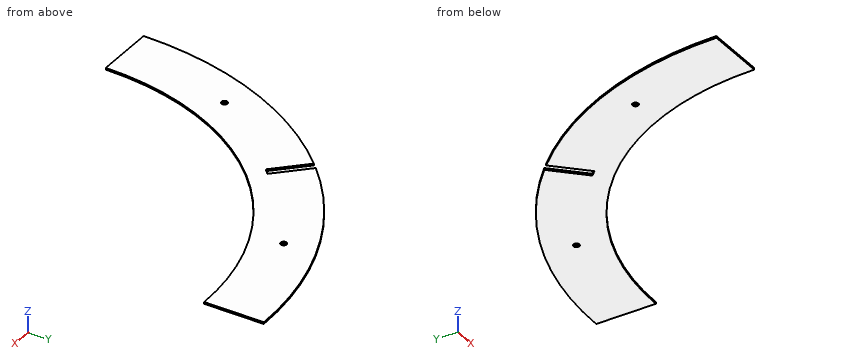
Autodesk Inventor part; units mm, degrees
ref_plane "YZ Plane" through (0, 0, 0) normal (1, 0, 0) x (0, 1, 0)
ref_plane "XZ Plane" through (0, 0, 0) normal (0, 1, 0) x (-1, 0, 0)
ref_plane "XY Plane" through (0, 0, 0) normal (0, 0, 1) x (1, 0, 0)
sketch "Sketch1" plane through (0, 0, 0) normal (0, 0, 1) x (1, 0, 0)
  arc A0 (0, 550) -> (-550, 0) centre (0, 0) ccw
  arc A1 (0, 450) -> (-450, 0) centre (0, 0) ccw
  line L0 (0, 550) -> (0, 450)
  line L1 (-450, 0) -> (-550, 0)
  point P0 (-500, 0)
  point P1 (0, 500)
  dimension "d0" = 1100
  dimension "d1" = 900
extrude "Plate1" add sketch "Sketch1" against normal blind 3
sketch "Sketch2" plane through (0, 0, 0) normal (0, 0, 1) x (1, 0, 0)
  line L0 (-550, 0) -> (-450, 0)
  arc A0 (0, 550) -> (-550, 0) centre (0, 0) ccw
  circle A1 centre (-461.9398, 191.3417) radius 5
  arc A2 (0, 450) -> (-450, 0) centre (0, 0) ccw
  line L1 (-415.7458, 172.2075) -> (-508.1337, 210.4759) construction
  point P0 (-461.9398, 191.3417)
  dimension "d4" = 10
  dimension "d5" = 22.5
extrude "Cut1" cut sketch "Sketch2" against normal through all
pattern_circular "Circular Pattern1" count 2 over 45 about axis through (0, 0, 0) along (0, 0, -1) of "Cut1"
sketch "Sketch3" plane through (0, 0, 0) normal (0, 0, 1) x (1, 0, 0)
  line L0 (-388.9087, 388.9087) -> (-318.1981, 318.1981) construction
  arc A0 (0, 450) -> (-450, 0) centre (0, 0) ccw
  arc A1 (0, 550) -> (-550, 0) centre (0, 0) ccw
  line L1 (-550, 0) -> (-450, 0)
  line L2 (-384.6661, 393.1514) -> (-393.1514, 384.6661)
  line L3 (-384.6661, 393.1514) -> (-335.1686, 343.6539)
  line L4 (-393.1514, 384.6661) -> (-343.6539, 335.1686)
  line L5 (-343.6539, 335.1686) -> (-335.1686, 343.6539)
  point P0 (-388.9087, 388.9087)
  dimension "d11" = 45
  dimension "d12" = 12
  dimension "d13" = 70
extrude "Extrusion1" cut sketch "Sketch3" against normal through all
equation "\"d0\" = Диаметр_вн"
equation "\"d1\" = d0 - 2 * Ширина_кольца"
equation "\"d4\" = Диаметр_отв"
equation "\"d6\" = Thickness"
equation "\"d2\" = Thickness"
equation "\"BendReliefWidth\" = Thickness"
equation "\"BendReliefDepth\" = 0.5 * Thickness"
equation "\"CornerReliefSize\" = 4 * Thickness"
equation "\"MinimumRemnant\" = 2 * Thickness"
equation "\"TransitionRadius\" = BendRadius"
equation "\"JacobiRadiusSize\" = BendRadius"
equation "\"GapSize\" = Thickness"
properties part number "BSH 502 segment" material "Stainless Steel"
Source: CAD feature listing. Evaluate the final solid. Frame: model axes, mm. Round coordinates to 2 decimals unless told otherwise and drop trailing zeros. Loops run counter-clockwise (first coordinate to the right, second up) from the corner with the lowest first, then second, coordinate; pieces in that order, holes last. Notation, with made-up numbers: (26, 0.25) - (37, 0.25) arc R16 cw to (37, 31.25) - close; hole circle Ø6 at (7.5, 29.5). An arc over 180 degrees is marked (long way). Write item = value, one per line. Start each with the question number.
(1) Pin query (flat end, axial travel): pin 1 (1 mm diameter, centred on y = 241, z = -1, fed in from -X). Return the tip coordinate at first contact, or that it passes through.
(2) Section query C-C, the plane y = 212. Output: boundary loops of the cut face in (x, z).
(3) Ray query, line 1 along Y through (x, z) = (-372, -0.3); line 2 along Y through (x, z) = (-379, -0.95); line 3 along X through (y, z) = (370.5, -0.15). Return the intervals inside material, ascending. Write a range as from..to.
(4) Section query D-D, the plane x = -516. Output: boundary loops of the cut face in (y, z).
(5) Section query B-B, the plane x = -358. Output: boundary loops of the cut face in (y, z), plus the area to 3 significant figures.
Conclusion:
q1.pin_1 = -494.63
q2.outline = (-507.5, -3) - (-396.93, -3) - (-396.93, 0) - (-507.5, 0) - close
q3.line_1 = 253.21..363.51, 380.49..405.11
q3.line_2 = 242.61..370.51, 387.49..398.57
q3.line_3 = -406.48..-378.99, -362.01..-255.4
q4.outline = (0, -3) - (190.38, -3) - (190.38, 0) - (0, 0) - close
q5.outline = (272.65, -3) - (349.51, -3) - (349.51, 0) - (272.65, 0) - close; (366.49, -3) - (417.54, -3) - (417.54, 0) - (366.49, 0) - close
q5.area = 384 mm2
